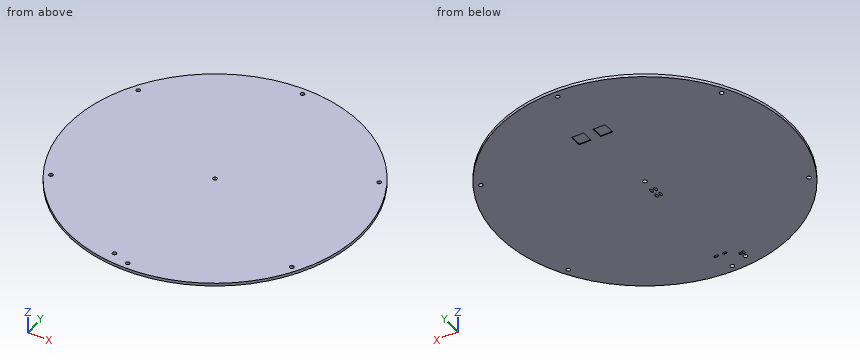
```python
from build123d import *

# Parameters (mm, degrees)
SKETCH1_R            = 110
BOSS_EXTRUDE1_DEPTH  = 2.2
SKETCH2_R            = 1.524
CUT_EXTRUDE1_DEPTH   = 156.579047432
CIRPATTERN1_COUNT    = 6
SKETCH3_W            = 9
SKETCH3_H            = 9
CUT_EXTRUDE2_DEPTH   = 0.5
SKETCH12_RX          = 1.807909399
SKETCH12_RY          = 1
CUT_EXTRUDE5_DEPTH   = 0.2
LPATTERN1_COUNT      = 2
LPATTERN1_PITCH      = 3
LPATTERN1_COUNT_DIR2 = 2
LPATTERN1_PITCH_DIR2 = 6.096
SKETCH13_R           = 1.524
CUT_EXTRUDE6_DEPTH   = 156.579047432
SKETCH14_RX          = 1.75
SKETCH14_RY          = 0.9
CUT_EXTRUDE7_DEPTH   = 0.2
LPATTERN2_COUNT      = 2
LPATTERN2_PITCH      = 6.4
SKETCH15_RX          = 1.441806236
SKETCH15_RY          = 0.830559885
SKETCH15_W           = 1.559100293
SKETCH15_H           = 2.883612472
CUT_EXTRUDE8_DEPTH   = 0.2


with BuildPart() as part:
    # Sketch1 → Boss-Extrude1 (new body)
    with BuildSketch(Plane.XY):
        Circle(SKETCH1_R)
    extrude(amount=BOSS_EXTRUDE1_DEPTH)

    # Sketch2 → Cut-Extrude1 (cut, through all)
    with BuildSketch(Plane.XY.offset(2.2)):
        with Locations((0, 105)):
            Circle(SKETCH2_R)
    cut_extrude1 = extrude(amount=-CUT_EXTRUDE1_DEPTH, mode=Mode.SUBTRACT)

    # CirPattern1: Cut-Extrude1 ×6 about axis
    cirpattern1_axis = Axis((0, 0, 0), (0, 0, 1))
    for i in range(1, CIRPATTERN1_COUNT):
        add(cut_extrude1.rotate(cirpattern1_axis, i * 360 / CIRPATTERN1_COUNT), mode=Mode.SUBTRACT)

    # Sketch3 → Cut-Extrude2 (cut)
    with BuildSketch(Plane(origin=(0, 0, 0), x_dir=(-1, 0, 0), z_dir=(0, 0, -1))):
        with Locations((-10.67, 59.436)):
            Rectangle(SKETCH3_W, SKETCH3_H)
        with Locations((5.588, 59.436)):
            Rectangle(SKETCH3_W, SKETCH3_H)
    extrude(amount=-CUT_EXTRUDE2_DEPTH, mode=Mode.SUBTRACT)

    # Sketch12 → Cut-Extrude5 (cut)
    with BuildSketch(Plane(origin=(0, 0, 0), x_dir=(-1, 0, 0), z_dir=(0, 0, -1))):
        with Locations(Location((-1.6002, -10.668), (0, 0, 90))):
            Ellipse(SKETCH12_RX, SKETCH12_RY)
    cut_extrude5 = extrude(amount=-CUT_EXTRUDE5_DEPTH, mode=Mode.SUBTRACT)

    # LPattern1: Cut-Extrude5 2 × 2
    with Locations(*[(-i * LPATTERN1_PITCH, -j * LPATTERN1_PITCH_DIR2, 0) for i in range(LPATTERN1_COUNT) for j in range(LPATTERN1_COUNT_DIR2) if (i, j) != (0, 0)]):
        add(cut_extrude5, mode=Mode.SUBTRACT)

    # Sketch13 → Cut-Extrude6 (cut, through all)
    with BuildSketch(Plane(origin=(0, 0, 0), x_dir=(-1, 0, 0), z_dir=(0, 0, -1))):
        Circle(SKETCH13_R)
        with Locations((12.7, -100.6602)):
            Circle(SKETCH13_R)
    extrude(amount=-CUT_EXTRUDE6_DEPTH, mode=Mode.SUBTRACT)

    # Sketch14 → Cut-Extrude7 (cut)
    with BuildSketch(Plane(origin=(0, 0, 0), x_dir=(-1, 0, 0), z_dir=(0, 0, -1))):
        with Locations(Location((-3.2, -90.805), (0, 0, 180))):
            Ellipse(SKETCH14_RX, SKETCH14_RY)
    cut_extrude7 = extrude(amount=-CUT_EXTRUDE7_DEPTH, mode=Mode.SUBTRACT)

    # LPattern2: Cut-Extrude7 ×2
    with Locations(*[(-i * LPATTERN2_PITCH, 0, 0) for i in range(1, LPATTERN2_COUNT)]):
        add(cut_extrude7, mode=Mode.SUBTRACT)

    # Sketch15 → Cut-Extrude8 (cut)
    with BuildSketch(Plane(origin=(0, 0, 0), x_dir=(-1, 0, 0), z_dir=(0, 0, -1))):
        with Locations(Location((11.398915538, -96.592408929), (0, 0, 90))):
            Ellipse(SKETCH15_RX, SKETCH15_RY)
        with Locations((13.804777386, -96.592408929)):
            Rectangle(SKETCH15_W, SKETCH15_H)
    extrude(amount=-CUT_EXTRUDE8_DEPTH, mode=Mode.SUBTRACT)


solid = part.part
```
For this review, take the finished solid that the model builds, in its own axes (mm). Give positions to 0.01 mm unless a question says otherwise; leave off trailing zeros. Write each loop counter-clockwise with the first axis right and the second up, starting at its lowest first coordinate (ties: lowest second). Pieces come first, ordered by that corner, then holes.
Item 1: Wall thickness on probe 1 along X at (y, z) = (51.5, 1.1); probe 2 along Y at (x, z) = (64, 0.9); probe 3 along Y at (x, z) = (-12.7, 1.7): over which ranges is each line inside the solid? List them lowest first.
Item 2: Take a section at B-B (x = 58.5). Give the boundary of the cut face in (y, z), and give its area (3 significant figures).
Item 3: Take a section at A-A (z = 0.95). Give the number of separate pieces and of enclosed holes in the cut face, and give its area (3 significant figures).
Item 4: Insertion check: P1, Ø0.9, axis at x = 3, y = -91, coming from the -Z side; P2, Ø1, axis at x = -24, z = 1.5, coming from the -Y side. Each pin has a flat end and moves straight along its axis. Give the tip position at first contact, or say it passes through.
Item 5: Take a section at C-C (y = -79.5). Give the boundary of the cut face in (x, z), and give its area (3 significant figures).
Established:
1. probe 1: x = -97.2 to -92.08, -89.78 to 89.78, 92.08 to 97.2
1. probe 2: y = -89.47 to 89.47
1. probe 3: y = -109.26 to -102.18, -99.14 to 109.26
2. outline: (-93.15, 0) - (93.15, 0) - (93.15, 2.2) - (-93.15, 2.2) - close
2. area: 410 mm2
3. separate pieces: 1
3. enclosed holes: 8
3. area: 38,000 mm2
4. P1: stops at z = 0.2
4. P2: stops at y = -107.46
5. outline: (-76.02, 0) - (76.02, 0) - (76.02, 2.2) - (-76.02, 2.2) - close
5. area: 335 mm2
